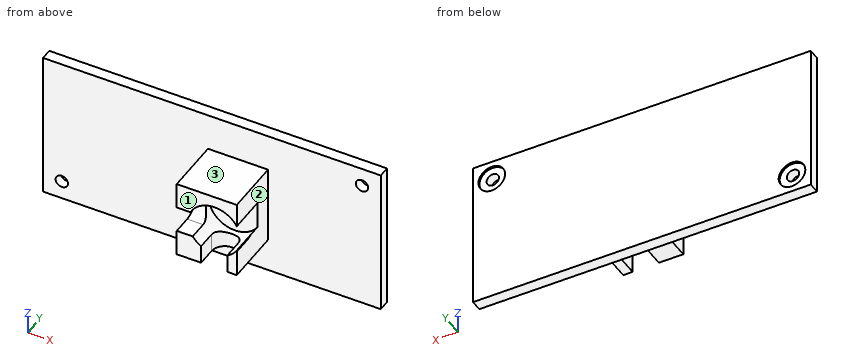
Solid Edge part; units mm, degrees
sketch "Sketch1" plane through (0, 0, 0) normal (0, -1, 0) x (1, 0, 0)
  line L0 (21.2, 4.4667) -> (41.2, 4.4667)
  line L1 (41.2, 4.4667) -> (41.2, 44.4667)
  line L2 (41.2, 44.4667) -> (21.2, 44.4667)
  line L3 (21.2, 44.4667) -> (21.2, 4.4667)
  dimension "D1" = 21.2
  dimension "D2" = 41.2
extrude "Protrusion1" add sketch "Sketch1" against normal blind 15
sketch "Sketch2" plane through (31.2, 0, 24.4667) normal (0, -1, 0) x (1, 0, 0)
  circle A0 centre (0, 10) radius 7
extrude "ExtrudedCutout_1" cut sketch "Sketch2" against normal blind 10
sketch "Sketch3" plane through (21.2, 7.5, 24.4667) normal (-1, 0, 0) x (0, -1, 0)
  line L0 (7.5, 13) -> (2.5, 13)
  arc A0 (2.5, 13) -> (2.5, 6) centre (2.5, 9.5) ccw
  line L1 (2.5, 6) -> (7.5, 6)
  line L2 (7.5, 13) -> (7.5, 6)
  dimension "D1" = 7.5
extrude "Cutout1" cut sketch "Sketch3" against normal through all
sketch "Sketch4" plane through (31.2, 15, 24.4667) normal (0, 1, 0) x (-1, 0, 0)
  line L0 (-10, 20) -> (-6, 20)
  line L1 (-6, 20) -> (-6, -20)
  line L2 (-6, -20) -> (-10, -20)
  line L3 (-10, -20) -> (-10, 20)
  dimension "D1" = 10
extrude "Cutout2" cut sketch "Sketch4" against normal through all
sketch "Sketch5" plane through (28.2, 7.5, 4.4667) normal (0, 0, -1) x (1, 0, 0)
  line L0 (6.5, 7.5) -> (6.5, 2.5)
  arc A0 (6.5, 2.5) -> (-0.5, 2.5) centre (3, 2.5) cw
  line L1 (-0.5, 2.5) -> (-0.5, 7.5)
  line L2 (6.5, 7.5) -> (-0.5, 7.5)
  dimension "D1" = 0.5
  dimension "D2" = 6.5
extrude "Cutout3" cut sketch "Sketch5" against normal up to next
sketch "Sketch6" plane through (28.2, 15, 24.4667) normal (0, 1, 0) x (-1, 0, 0)
  line L0 (-9, -20) -> (7, -20)
  line L1 (7, -20) -> (7, -1)
  line L2 (7, -1) -> (-9, -1)
  line L3 (-9, -1) -> (-9, -20)
  dimension "D1" = 7
extrude "Cutout4" cut sketch "Sketch6" against normal up to next
sketch "Sketch7" plane through (28.2, 15, 33.9667) normal (0, 1, 0) x (-1, 0, 0)
  line L0 (-39.04, 20.5) -> (-39.04, -19.5)
  line L1 (-39.04, -19.5) -> (50.96, -19.5)
  line L2 (50.96, 20.5) -> (50.96, -19.5)
  line L3 (-39.04, 20.5) -> (50.96, 20.5)
  dimension "D1" = 39.04
  dimension "D2" = 39.04
  dimension "D3" = 50.96
extrude "ExtrudedProtrusion_2" add sketch "Sketch7" along normal blind 3
sketch "Sketch8" plane through (19.24, 18, 34.4667) normal (0, 1, 0) x (-1, 0, 0)
  circle A0 centre (-43, 15) radius 1.65
  circle A1 centre (37, -15) radius 1.65
  dimension "D1" = 43
extrude "Cutout5" cut sketch "Sketch8" against normal through all
sketch "Sketch9" plane through (19.24, 18, 34.4667) normal (0, 1, 0) x (-1, 0, 0)
  circle A0 centre (-43, 15) radius 3.55
  circle A1 centre (37, -15) radius 3.55
extrude "ExtrudedCutout_9" cut sketch "Sketch9" against normal blind 0.5
Geometry: final body of the model. Coordinates: model frame, mm. Face numbers are marked on the shaded views. A direction names the side the tool comes from. Round coordinates to 2 decimals unless told otherwise and drop trailing zeros. Loops run counter-clockwise (first coordinate to the right, second up) from the corner with the lowest first, then second, coordinate; pieces in that order, holes last. Notation, with made-up numbers: M -22,87.5 L 10,87.5 A14 ccw 10,92.5 Z; hole C -11.5,50 d1. An arc over 180 degrees is marked long. Put each result on its own line as item: value. Start each with the question number.
(1) Contact query for flat-ended pins moving along their axis: pin 1 Ø4.5 at (x, z) = (62.24, 49.47) entering from +Y; pin 2 Ø5.5 at (y, z) = (2.5, 27) entering from -X; pin 3 Ø1.5 at (y, z) = (3, 26.5) entering from +X; pin 4 Ø8 at (x, y) = (13.5, 9.5) entering from +Z. Output: stop coordinate, or through.
(2) Set-up query: the marked faces 1, 2 and 3. Return all of +Z, -Z, +X, -X, +Y, -Y with unobstructed straight access to the full face (end or side cutting, diameter ignored); none if empty.
(3) Section query A-A (x = -17.76). Return loops of the section in (y, z).
(4) Section query B-B (y = 1.5). Return loops of the section in (x, z), then the cut area to 3 significant figures.
(5) Material intervals for line 1 along Z through (x, y) = (62.24, 17.8); line 2 along Z through (x, y) = (24.5, 2); line 3 along X through (y, z) = (14.5, 24), sorted ascending. Write a range as [from, to].
(6) Section query C-C (x = 31.2). Return loops of the section in (y, z), then the cut area to 3 significant figures.
(7) Section query D-D (y = 12.25). Return loops of the section in (x, z).
Findings below:
1. pin 1: stops at y = 17.5
1. pin 2: stops at x = 21.2
1. pin 3: stops at x = 37.2
1. pin 4: passes through
2. face 1: +Z, -Z, +X, -X, -Y
2. face 2: +Z, -Z, +X, -Y
2. face 3: +Z, +X, -X, -Y
3. outline: M 15,14.47 L 18,14.47 L 18,15.92 L 17.5,15.92 L 17.5,17.82 L 15,17.82 Z; M 15,21.12 L 17.5,21.12 L 17.5,23.02 L 18,23.02 L 18,54.47 L 15,54.47 Z
4. outline: M 21.2,23.47 L 27.7,23.47 L 27.7,28.4 A7 cw 25.46,30.47 L 21.2,30.47 Z; M 21.2,37.47 L 24.88,37.47 A7 cw 37.2,38.07 L 37.2,44.47 L 21.2,44.47 Z; M 34.7,23.47 L 37.2,23.47 L 37.2,30.47 L 36.94,30.47 A7 cw 34.7,28.4 Z
4. area: 133 mm2
5. line 1: z = [14.47, 45.92], [53.02, 54.47]
5. line 2: z = [23.47, 30.47], [37.47, 44.47]
5. line 3: x = [21.2, 37.2]
6. outline: M 0,41.47 L 10,41.47 L 10,27.47 L 8.5,27.47 L 8.5,23.47 L 15,23.47 L 15,14.47 L 18,14.47 L 18,54.47 L 15,54.47 L 15,44.47 L 0,44.47 Z
6. area: 261 mm2
7. outline: M 21.2,23.47 L 37.2,23.47 L 37.2,44.47 L 21.2,44.47 Z
